```python
from build123d import *

# Parameters (mm, degrees)
DOME1_FACE_RADIUS       = 2
DOME1_HEIGHT            = 2
SKETCH5_R               = 0.5
CUT_EXTRUDE1_DEPTH      = 4
SKETCH6_R               = 0.625
SKETCH6_R_2             = 0.5
EXTRUDE_THIN1_DEPTH     = 40
SKETCH7_R               = 9.506624516
CUT_EXTRUDE2_DEPTH      = 6
CUT_EXTRUDE2_DEPTH_BACK = 6


with BuildPart() as part:
    # Sketch2 → Revolve1 (revolve)
    with BuildSketch(Plane.XY):
        with BuildLine():
            Line((0, 0), (-1, 0))
            Line((-1, 0), (-1, 1.382676537))
            Line((-1, 1.382676537), (-14, 3.202544081))
            Line((-14, 3.202544081), (-14, 3.240195922))
            Line((-14, 3.240195922), (-14, 5))
            Line((-14, 5), (-13.5, 5))
            Line((-13.5, 5), (-13.5, 3.889862449))
            Line((-13.5, 3.889862449), (-10.3, 3.441895054))
            Line((-10.3, 3.441895054), (-10.3, 4.2))
            ThreePointArc((-10.3, 4.2), (-9.8, 4.7), (-9.3, 4.2))
            Line((-9.3, 4.2), (-9.3, 3.301905243))
            Line((-9.3, 3.301905243), (-8.3, 3.161915432))
            Line((-8.3, 3.161915432), (-8.3, 4))
            ThreePointArc((-8.3, 4), (-7.8, 4.5), (-7.3, 4))
            Line((-7.3, 4), (-7.3, 3.021925621))
            Line((-7.3, 3.021925621), (0, 2))
            Line((0, 2), (0, 0))
        make_face()
    revolve(axis=Axis((-26.179667308, 0, 0), (1, 0, 0)))

    # Dome1: a dome of height H over a round flat face of radius A is a cap of a sphere of radius (A * A + H * H) / (2 * H)
    dome1_r = (DOME1_FACE_RADIUS * DOME1_FACE_RADIUS + DOME1_HEIGHT * DOME1_HEIGHT) / (2 * DOME1_HEIGHT)
    dome1_base = Plane((0, 0, 0), z_dir=(1, 0, 0))
    with Locations(dome1_base.offset(DOME1_HEIGHT - dome1_r)):
        dome1_ball = Sphere(dome1_r, mode=Mode.PRIVATE)
    add(split(dome1_ball, bisect_by=dome1_base, keep=Keep.TOP, mode=Mode.PRIVATE))

    # Sketch5 → Cut-Extrude1 (cut, through all)
    with BuildSketch(Plane.ZY.offset(1)):
        Circle(SKETCH5_R)
    extrude(amount=-CUT_EXTRUDE1_DEPTH, mode=Mode.SUBTRACT)

    # Sketch6 → Extrude-Thin1 (add)
    with BuildSketch(Plane.ZY.offset(1)):
        Circle(SKETCH6_R)
        Circle(SKETCH6_R_2, mode=Mode.SUBTRACT)
    extrude(amount=-EXTRUDE_THIN1_DEPTH)

    # Sketch7 → Cut-Extrude2 (cut, two sides)
    with BuildSketch(Plane(origin=(0, 0, 0), x_dir=(1, 0, 0), z_dir=(0, 1, 0))) as cut_extrude2_sk:
        with Locations((39, 7.04259074)):
            Circle(SKETCH7_R)
    extrude(amount=CUT_EXTRUDE2_DEPTH, mode=Mode.SUBTRACT)
    extrude(cut_extrude2_sk.sketch, amount=-CUT_EXTRUDE2_DEPTH_BACK, mode=Mode.SUBTRACT)


solid = part.part
```
Can you work these out from the model? Positions are in its coordinate system, mm. A direction names the side the tool comes from. Round coordinates to 2 decimals unless told otherwise and drop trailing zeros. Loops run counter-clockwise (first coordinate to the right, second up) from the corner with the lowest first, then second, coordinate; pieces in that order, holes last.
Item 1: Which directions (+Z, -Z, +X, -X, +Y, -Y) give clear straight access to the entire face, cutting with the end or side of a thin tool? Please do faces 4 (the conical face through (-11.522, -0.783, -3.527)), 5 (the cylindrical face through (-13.75, -1.08, -4.88)), 6 (the flat face through (-7.3, -2, 3)).
Item 2: Please list where these lines run through material, in increasing order: L1, parallel to X at y = 1, z = 4.25; L2, parallel to X at y = 2.5, z = 3.5; L3, parallel to X at y = 1, z = -4.5.
Item 3: Will these pins go through, and if not, where does the flat tip stop? pin 1 Ø3 at (y, z) = (2.5, 1.5) entering from +X; pin 2 Ø1 at (x, z) = (3, 1.5) entering from +Y; pin 3 Ø6 at (x, z) = (3.5, -0.5) entering from +Y; pin 4 Ø2 at (y, z) = (3.5, 3) entering from +X.
Item 4: Suppose I cut it at A-A, the plane x = 6.5. Write out the boundary of the cut face in (y, z) (3 decimals), then the cut area to 3 significant figures.
Item 5: Suppose I cut it at B-B, the plane x = 0.5. Write out the boundary of the cut face in (y, z).
Item 6: If we mould it in two halves opening along Y, with no side actions, what happens to faces 1 (the flat face through (-13.5, 3, -3)), 2 (the flat face through (-1, 0, -1)), 3 (the conical face through (-3.6, -2.5, 0.1))? For each: +Y half, -Y half, draft (parallel to the pull), parting line (faces both ways), or undercut.
Reported:
1. face 4: none
1. face 5: +X, -X
1. face 6: +X
2. L1: x = -14 to -13.5, -10.27 to -9.33, -8.14 to -7.46
2. L2: x = -14 to -13.5, -10.29 to -9.31, -8.2 to -7.4
2. L3: x = -14 to -13.5, -10.09 to -9.51
3. pin 1: stops at x = 1.41
3. pin 2: passes through
3. pin 3: stops at y = 1.93
3. pin 4: stops at x = -7.3
4. outline: circle Ø1.25 at (0, 0); hole circle Ø1 at (0, 0)
4. area: 0.442 mm2
5. outline: circle Ø3.87 at (0, 0); hole circle Ø1 at (0, 0)
6. face 1: draft
6. face 2: undercut
6. face 3: parting line
